```python
from build123d import *

# Parameters (mm, degrees)
SKETCH_1_R          = 5
EXTRUDE_1_DEPTH     = 210
SHELL_1_T           = -1
CUT_EXTRUDE_1_REACH = 211.12
SKETCH_2_R          = 4


with BuildPart() as part:
    # 草图1 → 凸台-拉伸1 (new body)
    with BuildSketch(Plane.XY):
        Circle(SKETCH_1_R)
    extrude(amount=EXTRUDE_1_DEPTH)

    # 抽壳1
    shell_1_openings = [part.faces().sort_by_distance(p)[0] for p in [
        (0, 0, 210),
    ]]
    offset(amount=SHELL_1_T, openings=shell_1_openings, kind=Kind.INTERSECTION)

    # 草图2 → 切除-拉伸1 (cut, up to next)
    with BuildSketch(Plane.XY.offset(1), mode=Mode.PRIVATE) as cut_extrude_1_sk1:
        Circle(SKETCH_2_R)
    cut_extrude_1_tool1 = extrude(cut_extrude_1_sk1.sketch, amount=-CUT_EXTRUDE_1_REACH, mode=Mode.PRIVATE) & part.part
    add(cut_extrude_1_tool1.solids().sort_by_distance((0, 0, 1))[0], mode=Mode.SUBTRACT)


solid = part.part
```
CAD build for the part. Positions are in the model's coordinates, mm. Round coordinates to 2 decimals unless told otherwise and drop trailing zeros. Order: outer loops, then holes, each group sorted by start corner. A loop starts at its lowest first (then second) coordinate and runs counter-clockwise, first axis right, second up.
Q1. Wall check: L1, parallel to Y at x = 0.5, z = 59; L2, parallel to X at y = 1.5, z = 201; L3, parallel to X at y = 3.5, z = 109.5. Give the ranges that are in metal, low to high.
Q2. Slice it at A-A (y = 0). Write the cut outline in (x, z), and give its area (3 significant figures).
Q3. Drop flat-ended pins along their axis: pin 1 (2 mm diameter, centred on y = -2.5, z = 57.5, fed in from -X); pin 2 (2 mm diameter, centred on x = 2, y = 2, fed in from -Z). Give the stop position or say it passes through.
Results below:
1. L1: y = -4.97 to -3.97, 3.97 to 4.97
1. L2: x = -4.77 to -3.71, 3.71 to 4.77
1. L3: x = -3.57 to -1.94, 1.94 to 3.57
2. outline: (-5, 0) - (-4, 0) - (-4, 210) - (-5, 210) - close; (4, 0) - (5, 0) - (5, 210) - (4, 210) - close
2. area: 420 mm2
3. pin 1: stops at x = -4.77
3. pin 2: passes through
